Verification items for the finished model (mm, model axes). A direction names the side the tool comes from. Round coordinates to 2 decimals unless told otherwise and drop trailing zeros. Write each loop counter-clockwise with the first axis right and the second up, starting at its lowest first coordinate (ties: lowest second). Pieces come first, ordered by that corner, then holes. Notation, with made-up numbers: M 23,80.25 L 67,80.25 A31 ccw 67,110.25 Z; hole C 56.5,49.5 d6. An arc over 180 degrees is marked long. One line per item, written item: value. Start each with the question number.
from build123d import *

# Parameters (mm, degrees)
PAD_DEPTH              = 65
POCKET_DEPTH           = 65.001
SKETCH002_R            = 4
POCKET001_DEPTH        = 65.001
LINEARPATTERN_COUNT    = 6
LINEARPATTERN_PITCH    = 28
SKETCH003_W            = 170
SKETCH003_H            = 50
POCKET002_DEPTH        = 45
SKETCH004_W            = 30
SKETCH004_H            = 65
POCKET003_DEPTH        = 5
SKETCH005_R            = 3
POCKET004_DEPTH        = 50.001
SKETCH035_R            = 10
POCKET023_DEPTH        = 55.001
LINEARPATTERN001_COUNT = 3
LINEARPATTERN001_PITCH = 32.5


with BuildPart() as part:
    # Sketch → Pad (new body)
    with BuildSketch(Plane.XZ):
        Polygon((-9.174668, 84.617545), (30.825332, 84.617545), (30.825332, -85.382455), (-9.174668, -85.382455), (-24.174668, -70.382455), (-24.174668, 69.617545), align=None)
    extrude(amount=PAD_DEPTH)

    # Sketch001 (on Face8 of Pad) → Pocket (cut, through all)
    with BuildSketch(Plane.XZ.offset(65)):
        with BuildLine():
            ThreePointArc((0.825332, 70), (-4.174668, 75), (-9.174668, 70))
            Line((-9.174668, 70), (-9.174668, -70))
            ThreePointArc((-9.174668, -70), (-4.174668, -75), (0.825332, -70))
            Line((0.825332, 70), (0.825332, -70))
        make_face()
    extrude(amount=-POCKET_DEPTH, mode=Mode.SUBTRACT)

    # Sketch002 (on Face5 of Pocket) → Pocket001 (cut, through all)
    with BuildSketch(Plane.XZ.offset(65)):
        with Locations((10.825332, 69.617545)):
            Circle(SKETCH002_R)
    pocket001 = extrude(amount=-POCKET001_DEPTH, mode=Mode.SUBTRACT)

    # LinearPattern: Pocket001 ×6
    with Locations(*[(0, 0, -i * LINEARPATTERN_PITCH) for i in range(1, LINEARPATTERN_COUNT)]):
        add(pocket001, mode=Mode.SUBTRACT)

    # Sketch003 (on Face1 of LinearPattern) → Pocket002 (cut)
    with BuildSketch(Plane(origin=(-24.174668, 0, 0), x_dir=(0, 0, -1), z_dir=(-1, 0, 0))):
        with Locations((0.382455, 32.5)):
            Rectangle(SKETCH003_W, SKETCH003_H)
    extrude(amount=-POCKET002_DEPTH, mode=Mode.SUBTRACT)

    # Sketch004 (on Face8 of Pocket002) → Pocket003 (cut)
    with BuildSketch(Plane(origin=(30.825332, 0, 0), x_dir=(0, 0, 1), z_dir=(1, 0, 0))):
        with Locations((-70.382455, 32.5)):
            Rectangle(SKETCH004_W, SKETCH004_H)
        with Locations((69.617545, 32.5)):
            Rectangle(SKETCH004_W, SKETCH004_H)
    extrude(amount=-POCKET003_DEPTH, mode=Mode.SUBTRACT)

    # Sketch005 → Pocket004 (cut, through all)
    with BuildSketch(Plane(origin=(25.825332, 0, 0), x_dir=(0, 0, 1), z_dir=(1, 0, 0))):
        with Locations((-70.382455, 17.5)):
            Circle(SKETCH005_R)
        with Locations((-70.382455, 47.5)):
            Circle(SKETCH005_R)
        with Locations((69.617545, 47.5)):
            Circle(SKETCH005_R)
        with Locations((69.617545, 17.5)):
            Circle(SKETCH005_R)
    extrude(amount=-POCKET004_DEPTH, mode=Mode.SUBTRACT)

    # Sketch035 → Pocket023 (cut, through all)
    with BuildSketch(Plane(origin=(30.825332, 0, 0), x_dir=(0, 0, 1), z_dir=(1, 0, 0))):
        with Locations((-31.789585, 32.5)):
            Circle(SKETCH035_R)
    pocket023 = extrude(amount=-POCKET023_DEPTH, mode=Mode.SUBTRACT)

    # LinearPattern001: Pocket023 ×3
    with Locations(*[(0, 0, i * LINEARPATTERN001_PITCH) for i in range(1, LINEARPATTERN001_COUNT)]):
        add(pocket023, mode=Mode.SUBTRACT)


solid = part.part
1) Access from +Z, -Z, +X, -X, +Y, -Y to the whole of each face (thin tool, end or side, straight path). Record for faces 1 (the flat face through (25.825, -33, -71)), 2 (the flat face through (0.825, -4, 1)), 3 (the flat face through (3, -57.5, 1)), 4 (the flat face through (28, -32, 54.618)), 5 (the flat face through (-24.175, -4, -1)).
2) Cross-section at A-A (x = 17). Record the boundary of the cut face in (y, z).
3) Cross-section at B-B (y = -17.5). Record the boundary of the cut face in (x, z).
4) Thickness scan on line 1 (Z direction, x = 24.15, y = -47.5); line 2 (Y direction, x = 8.5, z = 73); line 3 (Z direction, x = 26.5, y = -45.5). Record the ranges inside material, lowest first.
5) Gauge pin test, flat ends, axial feed: pin 1 Ø6.5 at (x, z) = (10.83, 69.62) entering from +Y; pin 2 Ø1.5 at (x, y) = (29, -42) entering from -Z; pin 3 Ø8 at (y, z) = (-36.5, 25.5) entering from +X; pin 4 Ø10 at (y, z) = (-42, -20.5) entering from -X. Record the tip position at first contact, or that the pin passes through.
6) Cross-section at C-C (z = -25.5). Record the boundary of the cut face in (x, y), then the cut area to 3 significant figures.
7) Mould release check, pull along Y, two halves, no side actions. Record for faces 6 (the flat face through (-16.57, -61.198, -77.987)), 7 (the cylindrical face through (25.9, -22.74, -1.46)): pulls with the +Y half, pulls with the -Y half, needs draft (parallel to the pull), parting line crosses it, or undercut.
8) Cross-section at D-D (y = -59.5). Record the boundary of the cut face in (x, z), then the cut area to 3 significant figures.
Results below:
1. face 1: -Z, +X, +Y, -Y
1. face 2: +Y, -Y
1. face 3: +Z, -Z, -X
1. face 4: +Z, +X, +Y, -Y
1. face 5: +Z, -Z, -X, +Y, -Y
2. outline: M -65,-85.38 L -57.5,-85.38 L -57.5,84.62 L -65,84.62 Z; M -7.5,-85.38 L 0,-85.38 L 0,84.62 L -7.5,84.62 Z
3. outline: M 20.83,-85.38 L 25.83,-85.38 L 25.83,-73.38 L 20.83,-73.38 Z; M 20.83,-67.38 L 25.83,-67.38 L 25.83,-55.38 L 30.83,-55.38 L 30.83,54.62 L 25.83,54.62 L 25.83,66.62 L 20.83,66.62 Z; M 20.83,72.62 L 25.83,72.62 L 25.83,84.62 L 20.83,84.62 Z
4. line 1: z = -85.38 to -73.38, -67.38 to 66.62, 72.62 to 84.62
4. line 2: y = -65 to -57.5, -7.5 to 0
4. line 3: z = -55.38 to 54.62
5. pin 1: passes through
5. pin 2: stops at z = -55.38
5. pin 3: stops at x = 30.83
5. pin 4: stops at x = 20.83
6. outline: M -24.17,-65 L -9.17,-65 L -9.17,-57.5 L -24.17,-57.5 Z; M -24.17,-7.5 L -9.17,-7.5 L -9.17,0 L -24.17,0 Z; M 0.83,-65 L 30.83,-65 L 30.83,-40.27 L 20.83,-40.27 L 20.83,-57.5 L 0.83,-57.5 Z; M 0.83,-7.5 L 20.83,-7.5 L 20.83,-24.73 L 30.83,-24.73 L 30.83,0 L 0.83,0 Z
6. area: 1,020 mm²
7. face 6: needs draft
7. face 7: undercut
8. outline: M -24.17,-70.38 L -9.17,-85.38 L 25.83,-85.38 L 25.83,-55.38 L 30.83,-55.38 L 30.83,54.62 L 25.83,54.62 L 25.83,84.62 L -9.17,84.62 L -24.17,69.62 Z; hole M -9.17,-70 A5 ccw 0.83,-70 L 0.83,70 A5 ccw -9.17,70 Z; hole C 10.83,-70.38 d8; hole C 10.83,-42.38 d8; hole C 10.83,-14.38 d8; hole C 10.83,13.62 d8; hole C 10.83,41.62 d8; hole C 10.83,69.62 d8
8. area: 7,040 mm²
